Autodesk Fusion 360 part; units mm, degrees
sketch "Sketch1" plane through (0, 0, 0) normal (0, 0, 1) x (1, 0, 0)
  line L0 (0, 0) -> (26, 0)
  line L1 (26, 0) -> (26, 36)
  line L2 (26, 36) -> (0, 36)
  line L3 (0, 36) -> (0, 0)
  line L4 (3, 3) -> (23, 3)
  line L5 (3, 33) -> (3, 3)
  line L6 (23, 3) -> (23, 33)
  line L7 (23, 33) -> (3, 33)
  dimension "d2" = 30
sketch "Sketch3" plane through (0, 0, 0) normal (0, 0, 1) x (1, 0, 0)
  line L0 (12, 33) -> (14, 33)
  line L1 (14, 33) -> (14, 3)
  line L2 (14, 3) -> (12, 3)
  line L3 (12, 3) -> (12, 33)
  line L4 (23, 19) -> (3, 19)
  line L5 (3, 19) -> (3, 17)
  line L6 (3, 17) -> (23, 17)
  line L7 (23, 17) -> (23, 19)
extrude "Extrude1" add sketch "Sketch1" along normal blind 4
extrude "Extrude5" add sketch "Sketch3" along normal blind 4 contours L0 L1 L3 L4 | L1 L3 L4 L6 | L1 L2 L3 L6
extrude "Extrude6" add sketch "Sketch3" along normal blind 4 contours L3 L4 L5 L6
extrude "Extrude7" add sketch "Sketch3" along normal blind 4 contours L1 L4 L6 L7
sketch "Sketch5" plane through (0, 0, 0) normal (0, 0, 1) x (1, 0, 0)
  line L0 (26, 36) -> (0, 36)
  line L1 (0, 0) -> (26, 0)
  line L2 (0, 36) -> (0, 0)
  line L3 (26, 0) -> (26, 36)
extrude "Extrude9" add sketch "Sketch5" along normal blind 1
move_face "OffsetFaces1" offset -0.75 1 faces at (8.6667, 24, 0)
extrude "Extrude8" [suppressed]
extrude "Extrude4" [suppressed]
extrude "Extrude3" [suppressed]
extrude "Extrude2" [suppressed]
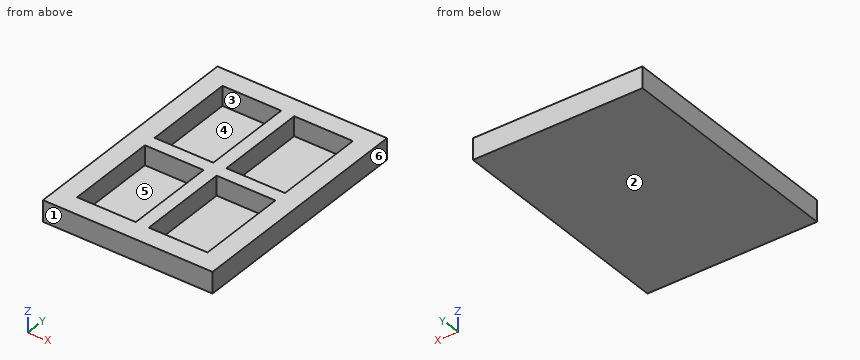
Here's how the part is built. I have some questions about the finished solid (model axes, mm). Face numbers are marked on the shaded views. A direction names the side the tool comes from. Round coordinates to 2 decimals unless told otherwise and drop trailing zeros. Write each loop counter-clockwise with the first axis right and the second up, starting at its lowest first coordinate (ties: lowest second). Pieces come first, ordered by that corner, then holes.
1. If we mould it in two halves opening along Y, with no side actions, what happens to the marked faces 1, 2, 3 and 4? For each: released by +Y, released by -Y, zero draft, split by the parting line, or undercut.
2. Will this pin go through, and if not, where does the flat tip stop? pin 1 Ø2.5 at (x, y) = (8.5, 10.5) entering from +Z.
3. I need wall thicknesses on L1, parallel to Y at x = 7.5, z = 3.55; L2, parallel to X at y = 6, z = 1.2; L3, parallel to Z at x = 18.5, y = 32.5. Which ranges of each line are inside material? Lowest first, please.
4. For the marked faces 5 and 6, which set-ups out of +Z, -Z, +X, -X, +Y, -Y let a thin tool reach every point of the face, with its end or its side?
5. Suppose I cut it at A-A (x = 4.5). List the corners of the cut face in (y, z) for me.
6. Suppose I cut it at B-B (z = 3.5). List the corners of the cut face in (x, y) for me.
7. Suppose I cut it at C-C (y = 28.5). List the corners of the cut face in (x, z) for me.
Answer sheet:
1. face 1: released by -Y
1. face 2: zero draft
1. face 3: undercut
1. face 4: undercut
2. pin 1: stops at z = 1
3. L1: y = 0 to 3, 17 to 19, 33 to 36
3. L2: x = 0 to 3, 12 to 14, 23 to 26
3. L3: z = 0.75 to 1
4. face 5: +Z
4. face 6: +Z, -Z, +X, +Y, -Y
5. outline: (0, 0.75) - (36, 0.75) - (36, 4) - (33, 4) - (33, 1) - (19, 1) - (19, 4) - (17, 4) - (17, 1) - (3, 1) - (3, 4) - (0, 4) - close
6. outline: (0, 0) - (26, 0) - (26, 36) - (0, 36) - close; hole (3, 3) - (12, 3) - (12, 17) - (3, 17) - close; hole (3, 19) - (12, 19) - (12, 33) - (3, 33) - close; hole (14, 3) - (23, 3) - (23, 17) - (14, 17) - close; hole (14, 19) - (23, 19) - (23, 33) - (14, 33) - close
7. outline: (0, 0.75) - (26, 0.75) - (26, 4) - (23, 4) - (23, 1) - (14, 1) - (14, 4) - (12, 4) - (12, 1) - (3, 1) - (3, 4) - (0, 4) - close
